Build history of the part. All positions in model axes, mm. Face numbers are marked on the shaded views. Give positions to 0.01 mm unless a question says otherwise; leave off trailing zeros. Put each result on its own line as item: value.
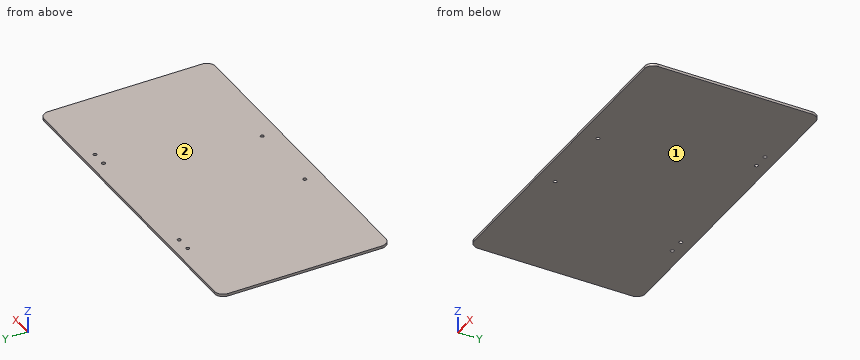
from build123d import *

# Parameters (mm, degrees)
SKETCH_1_W          = 380
SKETCH_1_H          = 200
EXTRUDE_1_DEPTH     = 3
SKETCH_2_R          = 2.075
CUT_EXTRUDE_1_DEPTH = 215.730063102
FILLET_1_R          = 10
SKETCH_3_R          = 2.075
CUT_EXTRUDE_2_DEPTH = 5


with BuildPart() as part:
    # 草图1 → 凸台-拉伸1 (new body)
    with BuildSketch(Plane.XY):
        Rectangle(SKETCH_1_W, SKETCH_1_H)
    extrude(amount=EXTRUDE_1_DEPTH)

    # 草图2 → 切除-拉伸1 (cut, through all)
    with BuildSketch(Plane.XY.offset(3)):
        with Locations((-98, 86)):
            Circle(SKETCH_2_R)
        with Locations((-80, 86)):
            Circle(SKETCH_2_R)
        with Locations(Location((80, 86, 0), (0, 0, 180))):
            Circle(SKETCH_2_R)
        with Locations(Location((98, 86, 0), (0, 0, 180))):
            Circle(SKETCH_2_R)
    extrude(amount=-CUT_EXTRUDE_1_DEPTH, mode=Mode.SUBTRACT)

    # 圆角1
    fillet_1_edges = [part.edges().sort_by_distance(p)[0] for p in [
        (190, -100, 1.5),
        (-190, -100, 1.5),
        (-190, 100, 1.5),
        (190, 100, 1.5),
    ]]
    fillet(fillet_1_edges, radius=FILLET_1_R)

    # 草图3 → 切除-拉伸2 (cut)
    with BuildSketch(Plane.XY.offset(3)):
        with Locations((-45, -80)):
            Circle(SKETCH_3_R)
        with Locations((45, -80)):
            Circle(SKETCH_3_R)
    extrude(amount=-CUT_EXTRUDE_2_DEPTH, mode=Mode.SUBTRACT)


solid = part.part
1) Wall check: L1, parallel to X at y = -80.5, z = 1.3; L2, parallel to Y at x = -80, z = 1 (3 decimals); L3, parallel to X at y = 92, z = 0.7. Give the ranges that are in metal, low to high.
Filled sheet:
L1: -190 to -47.01, -42.99 to 42.99, 47.01 to 190
L2: -100 to 83.925, 88.075 to 100
L3: -189.8 to 189.8
2) Pull direction Z, two halves, no side cores. Call the marked faces 1 and 2: released by +Z, released by -Z, zero draft, split by the parting line, or undercut.
Filled sheet:
face 1: released by -Z
face 2: released by +Z
3) Pin check, flat tips, straight feed: pin 1 (3.5 mm diameter, centred on x = -98, y = 86, fed in from -Z); pin 2 (5.5 mm diameter, centred on x = 45, y = -80, fed in from -Z). Stop position of each tip, or through.
Filled sheet:
pin 1: through
pin 2: z = 0
